Read the model definition and answer for the solid it produces. Units are mm, in the model's axes. Face numbers are marked on the shaded views. A direction names the side the tool comes from. Round coordinates to 2 decimals unless told otherwise and drop trailing zeros. Loops run counter-clockwise (first coordinate to the right, second up) from the corner with the lowest first, then second, coordinate; pieces in that order, holes last. Notation, with made-up numbers: (7, 75) -> (57, 75) arc R16 cw to (57, 83) -> close; hole circle Ø7 at (18, -30). An arc over 180 degrees is marked (long way). Put each result on its own line as item: value.
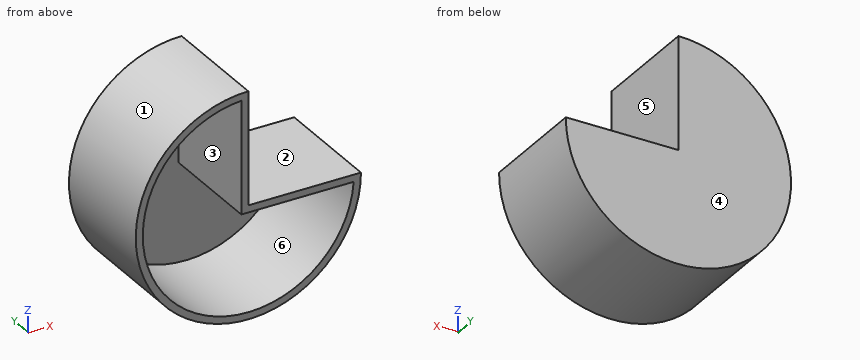
from build123d import *

# Parameters (mm, degrees)
BOSS_EXTRUDE1_DEPTH = 80
SHELL1_T            = -5


with BuildPart() as part:
    # Sketch2 → Boss-Extrude1 (new body)
    with BuildSketch(Plane(origin=(0, 0, 0), x_dir=(1, 0, 0), z_dir=(0, 1, 0))):
        with BuildLine():
            Line((0, 0), (80, 0))
            ThreePointArc((80, 0), (-56.568542495, 56.568542495), (0, -80))
            Line((0, -80), (0, 0))
        make_face()
    extrude(amount=BOSS_EXTRUDE1_DEPTH)

    # Shell1
    shell1_openings = [part.faces().sort_by_distance(p)[0] for p in [
        (-5.522847498, 0, -5.522847498),
    ]]
    offset(amount=SHELL1_T, openings=shell1_openings, kind=Kind.INTERSECTION)


solid = part.part
Item 1: Which of the six approach directions +Z, -Z, +X, -X, +Y, -Y give full straight-line access (tool end or side, diameter ignored) to the marked faces 4, 5 and 6?
Derived:
face 4: +Z, -Z, +X, -X, +Y
face 5: +Z, +X, +Y, -Y
face 6: -Y
Item 2: The part is cut by section B-B (x = -22). Determine the outline of the cut face in (y, z), then the cut area to 3 significant figures.
Derived:
outline: (0, -76.92) -> (80, -76.92) -> (80, 76.92) -> (0, 76.92) -> (0, 71.7) -> (75, 71.7) -> (75, -71.7) -> (0, -71.7) -> close
area: 1,550 mm^2
Item 3: Flat-ended cylindrical pins translate along their axes: pin 1 Ø12 at (x, y) = (-48, 50) entering from +Z; pin 2 Ø12 at (x, y) = (-30, 40.5) entering from +Z; pin 3 Ø1 at (y, z) = (47.5, -12) entering from -X. Find the tip coordinate at first contact, or state that the pin passes through.
Derived:
pin 1: stops at z = 68.09
pin 2: stops at z = 76.32
pin 3: stops at x = -79.17
Item 4: The part is cut by section A-A (y = 16). Determine the outline of the cut face in (x, z).
Derived:
outline: (0, 0) -> (0, 80) arc R80 ccw (long way) to (80, 0) -> close; hole (-5, -5) -> (-5, 74.83) arc R75 ccw (long way) to (74.83, -5) -> close
Item 5: For a pull along X with two mould halves and no side action, classify the marked faces 1, 2 and 3 as pulls with the +X half, pulls with the -X half, needs draft (parallel to the pull), parting line crosses it, or undercut.
Derived:
face 1: parting line crosses it
face 2: needs draft
face 3: undercut
Item 6: Find the intervals of material crossed by line 1 along Y through (x, z) = (42, -51); line 2 along Z through (x, y) = (-6, 19.5); line 3 along X through (y, z) = (37, -0.5), in increasing order.
Derived:
line 1: y = 75 to 80
line 2: z = -79.77 to -74.76, 74.76 to 79.77
line 3: x = -80 to -75, -5 to 80
Item 7: The part is cut by section C-C (z = -57.5). Determine the outline of the cut face in (x, y).
Derived:
outline: (-55.62, 0) -> (-48.15, 0) -> (-48.15, 75) -> (48.15, 75) -> (48.15, 0) -> (55.62, 0) -> (55.62, 80) -> (-55.62, 80) -> close
